For this review, take the finished solid that the model builds, in its own axes (mm). A direction names the side the tool comes from. Give positions to 0.01 mm unless a question says otherwise; leave off trailing zeros. Write each loop counter-clockwise with the first axis right and the second up, starting at its lowest first coordinate (ties: lowest second). Pieces come first, ordered by that corner, then holes.
1) Draft analysis for pull direction X (two halves, no side actions). For faces 1 (the face through (48, 0, 2)), 2 (the face through (98, 22, 2)), 3 (the face through (-22, 0, 2)), state which applies: pulls with the +X half, pulls with the -X half, needs draft (parallel to the pull), parting line crosses it, or undercut.
2) Wall thickness on line 1 along Y through (x, z) = (25, 3.5); line 2 along Y through (x, z) = (29, 3.05); line 3 along X through (y, z) = (9.5, 6.75): over which ranges is each line inside the solid? List them lowest first.
3) We need section C-C on y = 9. Give the boundary of the cut face in (x, z).
4) Machinability: for faces 4 (the face through (9.139, 14.334, 7.465)), 5 (the face through (216, 0, 2)), 6 (the face through (181, 4, 5)), which of the approach directions +Z, -Z, +X, -X, +Y, -Y give a long, thin tool a straight path to every point of the face, cutting with its end or side? Answer none if there is none.
5) We need section B-B on x = 127. Give the boundary of the cut face in (y, z).
6) For P1, Ø8, axis at x = 29, y = 0, coming from the +Z side; P2, Ø3.5, axis at x = 127, y = -18, coming from the -Z side; P3, Ø1.5, axis at y = -6, z = 2.5, coming from the -X side, all flat-tipped, find the tip position at first contact; note any pin that passes through.
7) We need section D-D on x = 46. Give the boundary of the cut face in (y, z), and give its area (3 significant figures).
8) We need section A-A on z = 8.25. Give the boundary of the cut face in (x, y), and give its area (3 significant figures).
from build123d import *

# Parameters (mm, degrees)
BOSS_EXTRUDE1_DEPTH     = 5
SKETCH2_R               = 17
SKETCH2_R_2             = 12
BOSS_EXTRUDE2_DEPTH     = 5
SKETCH3_R               = 12
CUT_EXTRUDE1_DEPTH      = 6
SKETCH5_R               = 2
SKETCH5_R_2             = 3.5
CUT_EXTRUDE2_DEPTH      = 10
SKETCH9_W               = 4
SKETCH9_H               = 8
CUT_EXTRUDE4_DEPTH      = 10
M2_5_TAPPED_HOLE1_D     = 2.05
M2_5_TAPPED_HOLE1_DEPTH = 5.734117865
M2_5_TAPPED_HOLE1_TIP   = 0.615882135


with BuildPart() as part:
    # Sketch1 → Boss-Extrude1 (new body)
    with BuildSketch(Plane.XY):
        with BuildLine():
            Line((194, 22), (0, 22))
            ThreePointArc((0, 22), (-22, 0), (0, -22))
            Line((0, -22), (194, -22))
            ThreePointArc((194, -22), (216, 0), (194, 22))
        make_face()
    extrude(amount=BOSS_EXTRUDE1_DEPTH)

    # Sketch2 → Boss-Extrude2 (add)
    with BuildSketch(Plane.XY.offset(5)):
        Circle(SKETCH2_R)
        Circle(SKETCH2_R_2, mode=Mode.SUBTRACT)
        with Locations((194, 0)):
            Circle(SKETCH2_R)
        with Locations((194, 0)):
            Circle(SKETCH2_R_2, mode=Mode.SUBTRACT)
    extrude(amount=BOSS_EXTRUDE2_DEPTH)

    # Sketch3 → Cut-Extrude1 (cut)
    with BuildSketch(Plane.XY.offset(5)):
        with Locations((194, 0)):
            Circle(SKETCH3_R)
        Circle(SKETCH3_R)
    extrude(amount=-CUT_EXTRUDE1_DEPTH, mode=Mode.SUBTRACT)

    # Sketch5 → Cut-Extrude2 (cut)
    with BuildSketch(Plane(origin=(0, 0, 0), x_dir=(-1, 0, 0), z_dir=(0, 0, -1))):
        with Locations((-169, 18)):
            Circle(SKETCH5_R)
        with Locations((-67, 18)):
            Circle(SKETCH5_R)
        with Locations((-67, -18)):
            Circle(SKETCH5_R)
        with Locations((-169, -18)):
            Circle(SKETCH5_R)
        with Locations((-127, 18)):
            Circle(SKETCH5_R)
        with Locations((-127, -18)):
            Circle(SKETCH5_R)
        with Locations((-25, 18)):
            Circle(SKETCH5_R)
        with Locations((-25, -18)):
            Circle(SKETCH5_R)
        with Locations((-148, 0)):
            Circle(SKETCH5_R)
        with Locations((-97, 0)):
            Circle(SKETCH5_R)
        with Locations((-46, 0)):
            Circle(SKETCH5_R)
        with Locations((-165, 0)):
            Circle(SKETCH5_R_2)
        with Locations((-29, 0)):
            Circle(SKETCH5_R_2)
    extrude(amount=-CUT_EXTRUDE2_DEPTH, mode=Mode.SUBTRACT)

    # Sketch9 → Cut-Extrude4 (cut)
    with BuildSketch(Plane(origin=(0, 0, 0), x_dir=(-1, 0, 0), z_dir=(0, 0, -1))):
        with Locations((-180.7, 0)):
            Rectangle(SKETCH9_W, SKETCH9_H)
    extrude(amount=-CUT_EXTRUDE4_DEPTH, mode=Mode.SUBTRACT)

    # M2.5 Tapped Hole1
    with Locations(Plane(origin=(0, 0, 0), x_dir=(-1, 0, 0), z_dir=(0, 0, -1))):
        with Locations((0, 14), (14, 0), (0, -14), (-14, 0)):
            Hole(M2_5_TAPPED_HOLE1_D / 2, depth=M2_5_TAPPED_HOLE1_DEPTH)
            with Locations((0, 0, -(M2_5_TAPPED_HOLE1_DEPTH + M2_5_TAPPED_HOLE1_TIP / 2))):  # 118° drill point
                Cone(0, M2_5_TAPPED_HOLE1_D / 2, M2_5_TAPPED_HOLE1_TIP, mode=Mode.SUBTRACT)


solid = part.part
Results list:
1. face 1: undercut
1. face 2: needs draft
1. face 3: pulls with the -X half
2. line 1: y = -22 to -20, -16 to 16, 20 to 22
2. line 2: y = -22 to -3.5, 3.5 to 22
2. line 3: x = -14.1 to -7.33, 7.33 to 14.1, 179.9 to 186.67, 201.33 to 208.1
3. outline: (-20.07, 0) - (-7.94, 0) - (-7.94, 10) - (-14.42, 10) - (-14.42, 5) - (-20.07, 5) - close; (7.94, 0) - (186.06, 0) - (186.06, 10) - (179.58, 10) - (179.58, 5) - (14.42, 5) - (14.42, 10) - (7.94, 10) - close; (201.94, 0) - (214.07, 0) - (214.07, 5) - (208.42, 5) - (208.42, 10) - (201.94, 10) - close
4. face 4: +Z
4. face 5: +Z, -Z, +X
4. face 6: +Z, -Z
5. outline: (-22, 0) - (-20, 0) - (-20, 5) - (-22, 5) - close; (-16, 0) - (16, 0) - (16, 5) - (-16, 5) - close; (20, 0) - (22, 0) - (22, 5) - (20, 5) - close
6. P1: stops at z = 5
6. P2: passes through
6. P3: stops at x = -21.36
7. outline: (-22, 0) - (-2, 0) - (-2, 5) - (-22, 5) - close; (2, 0) - (22, 0) - (22, 5) - (2, 5) - close
7. area: 200 mm2
8. outline: circle Ø34 at (0, 0); circle Ø34 at (194, 0); hole circle Ø24 at (0, 0); hole (178.7, -4) - (182.69, -4) arc R12 ccw (long way) to (182.69, 4) - (178.7, 4) - close
8. area: 883 mm2
